```python
from build123d import *

# Parameters (mm, degrees)
SKETCH1_R   = 1.4224
SHAFT_DEPTH = 25.4
SKETCH2_R   = 2.3241
HEAD_DEPTH  = 2.8448
FILLET1_R   = 0.254
HEX_2_DEPTH = 1.905


with BuildPart() as part:
    # Sketch1 → Shaft (new body)
    with BuildSketch(Plane(origin=(0, 0, 0), x_dir=(1, 0, 0), z_dir=(0, 1, 0))):
        with Locations(Location((0, 0, 0), (0, 0, 270))):
            Circle(SKETCH1_R)
    extrude(amount=-SHAFT_DEPTH)

    # Sketch2 → Head (add)
    with BuildSketch(Plane(origin=(0, 0, 0), x_dir=(1, 0, 0), z_dir=(0, 1, 0))):
        with Locations(Location((0, 0, 0), (0, 0, 270))):
            Circle(SKETCH2_R)
    extrude(amount=HEAD_DEPTH)

    # Fillet1
    fillet1_edges = [part.edges().sort_by_distance(p)[0] for p in [
        (0, 2.8448, -2.3241),
    ]]
    fillet(fillet1_edges, radius=FILLET1_R)

    # Sketch3 → Hex 2 (cut)
    with BuildSketch(Plane(origin=(0, 2.8448, 0), x_dir=(1, 0, 0), z_dir=(0, 1, 0))):
        Polygon((0, 1.374815329), (-1.190625, 0.687407664), (-1.190625, -0.687407664), (0, -1.374815329), (1.190625, -0.687407664), (1.190625, 0.687407664), align=None)
    extrude(amount=-HEX_2_DEPTH, mode=Mode.SUBTRACT)


solid = part.part
```
Source: CAD feature listing. Evaluate the final solid. Frame: model axes, mm. A direction names the side the tool comes from. Coordinates: 2 decimals unless noted, no trailing zeros. Order: outer loops, then holes, each group sorted by start corner. A loop starts at its lowest first (then second) coordinate and runs counter-clockwise, first axis right, second up. Notation, with made-up numbers: M 13,77 L 58,77 A27 cw 58,110 Z; hole C -17.75,11.25 d11. An arc over 180 degrees is marked long. Write each question's results on one line, items separated by ' | '. Start each with the question number.
1) Draft query along Z for faces 1 (the face through (0, 0.94, 0)), 2 (the face through (-1.39, -12.52, -0.31)), 3 (the face through (-2, 0, 0)). Return one class per face: released by +Z, released by -Z, zero draft, split by the parting line, or undercut.
2) Section query B-B (y = -8). Return the cut outline in (x, z), plus the area to 3 significant figures.
3) Contact query for a flat-ended pin moving along its axis: pin 1 Ø2 at (y, z) = (-18, 0) entering from +X. Output: stop coordinate, or through.
4) Section query A-A (z = 0). Return the cut outline in (x, y), plus the area to 3 significant figures.
5) Access query for faces 4 (the face through (-1.191, 2, 0)), 5 (the face through (-1, 2.845, 1)). Directions: +Z, -Z, +X, -X, +Y, -Y. A direction counts if a zero-diameter tool reaches every point of the face in a straight line with its end or side. Return the directions, or none.
6) Line query: line 1 (Y direction, x = -1.45, z = -1.55); line 2 (X direction, y = -15, z = 0.1); line 3 (Y direction, x = -1.15, z = 0.15). Output: solid intervals per line, ascending. Write a range as from..to.
Answers:
1) face 1: undercut | face 2: split by the parting line | face 3: zero draft
2) outline: C 0,0 d2.84 | area: 6.36 mm^2
3) pin 1: stops at x = 1.42
4) outline: M -2.32,0 L -1.42,0 L -1.42,-25.4 L 1.42,-25.4 L 1.42,0 L 2.32,0 L 2.32,2.59 A0.25 ccw 2.07,2.84 L 1.19,2.84 L 1.19,0.94 L -1.19,0.94 L -1.19,2.84 L -2.07,2.84 A0.25 ccw -2.32,2.59 Z | area: 80.9 mm^2
5) face 4: +Y | face 5: +Z, -Z, +X, -X, +Y
6) line 1: y = 0..2.84 | line 2: x = -1.42..1.42 | line 3: y = -25.4..0.94
